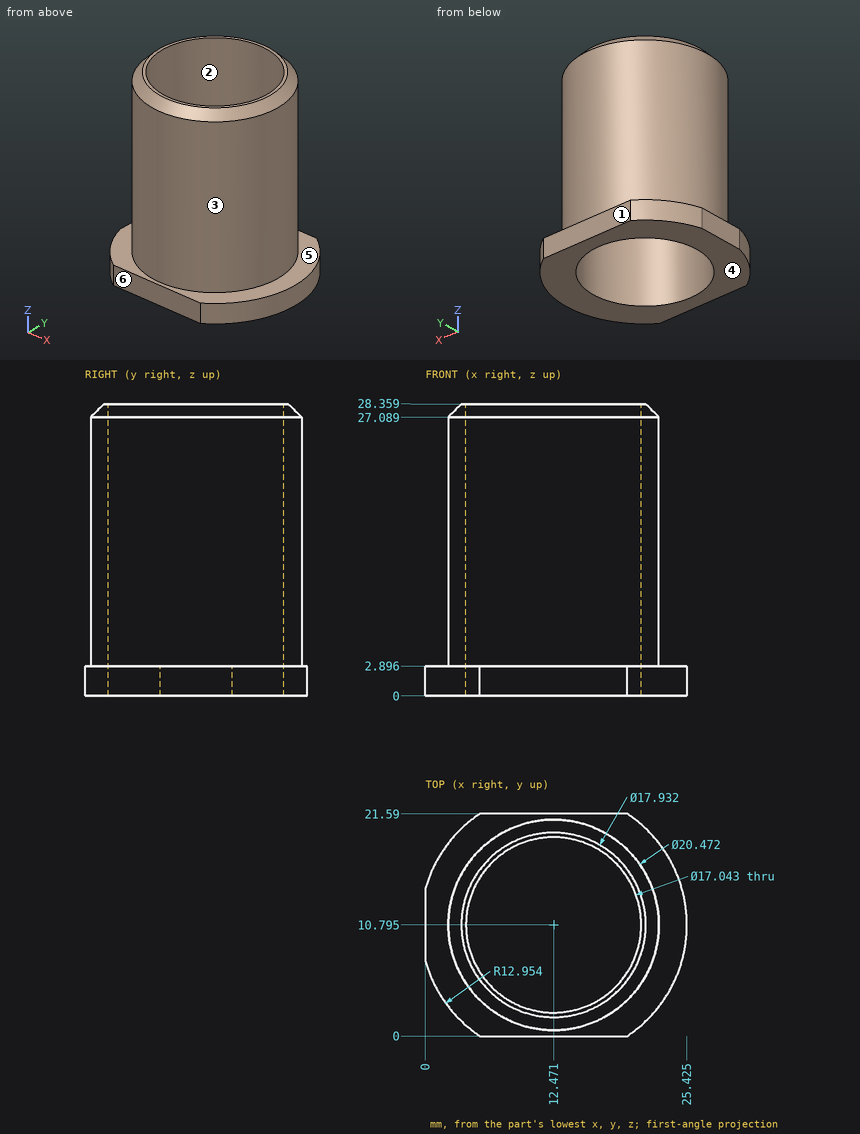
Answer from the drawing. Dimensions are ordinates in mm from the lowest x, y and z of the part. A direction names the side the tool comes from. Round coordinates to 2 decimals unless told otherwise and drop trailing zeros.
(1) Find the intervals of material crossed by L1, parallel to X at y = 18, z = 18 (1 decimal); L2, parallel to Z at x = 3, y = 17.75 (1 decimal); L3, parallel to Y at x = 10, z = 23.25, in increasing order.
Computed values:
L1: x = 5.2 to 7.9, 17 to 19.7
L2: z = 0 to 2.9
L3: y = 0.86 to 2.64, 18.95 to 20.73
(2) The mould has two halves that part along Y. Classify the marked faces 1, 2, 3 and 4: pulls with the +Y half, pulls with the -Y half, needs draft (parallel to the pull), parting line crosses it, or undercut.
Computed values:
face 1: pulls with the +Y half
face 2: undercut
face 3: parting line crosses it
face 4: needs draft
(3) Each of these flat-tipped pins is pushed along its axis until it touches: P1, Ø12, axis at y = 17.5, z = 8.5, coming from the -X side; P2, Ø8, axis at y = 17, z = 24.5, coming from the +X side; P3, Ø4, axis at x = 17, y = 10.5, coming from the -Z side; P4, Ø3, axis at y = 10.5, z = 16.5, coming from the -X side (1 decimal). Where does it stop, or does it pass through?
Computed values:
P1: stops at x = 0.35
P2: stops at x = 22.47
P3: passes through
P4: stops at x = 2.2
(4) For the marked faces 5 and 6, determine the directions among +Z, -Z, +X, -X, +Y, -Y from which every point of the face is accessible in a straight line to the end or side of a thin tool.
Computed values:
face 5: +Z
face 6: +Z, -Z, +X, -X, -Y
